from build123d import *

# Parameters (mm, degrees)
SKETCH_R     = 4
PAD_DEPTH    = 8
SKETCH001_R  = 2.85
PAD001_DEPTH = 9
SKETCH002_R  = 2.4
PAD002_DEPTH = 6
CHAMFER_SIZE = 1


with BuildPart() as part:
    # Sketch → Pad (new body)
    with BuildSketch(Plane.XY):
        Circle(SKETCH_R)
    extrude(amount=PAD_DEPTH)

    # Sketch001 (on Face3 of Pad) → Pad001 (join)
    with BuildSketch(Plane.XY.offset(8)):
        Circle(SKETCH001_R)
    extrude(amount=PAD001_DEPTH)

    # Sketch002 (on Face5 of Pad001) → Pad002 (join)
    with BuildSketch(Plane.XY.offset(17)):
        Circle(SKETCH002_R)
    extrude(amount=PAD002_DEPTH)

    # Chamfer
    chamfer_edges = [part.edges().sort_by_distance(p)[0] for p in [
        (-4, 0, 0),
    ]]
    chamfer(chamfer_edges, length=CHAMFER_SIZE)


solid = part.part
Part model, mm, in its own coordinate system. A direction names the side the tool comes from. Coordinates: 2 decimals unless noted, no trailing zeros. Order: outer loops, then holes, each group sorted by start corner. A loop starts at its lowest first (then second) coordinate and runs counter-clockwise, first axis right, second up. Notation, with made-up numbers: M 60.5,20.5 L 99.5,20.5 A22 cw 99.5,46.5 Z; hole C -21,33 d2. An arc over 180 degrees is marked long. Use a Markdown table: item, result.
(1) Probe L1, parallel to Z at x = -2, y = 1.5; L2, parallel to Y at x = -2.5, z = 5; L3, parallel to X at y = 0.5, z = 3. List the from-to ranges inside material, lowest first.
A:
| item | result |
|---|---|
| L1 | z = 0 to 17 |
| L2 | y = -3.12 to 3.12 |
| L3 | x = -3.97 to 3.97 |
(2) Flat gauge pins, fed straight in: pin 1 (4 mm diameter, centred on y = -1.5, z = 17, fed in from -X); pin 2 (3 mm diameter, centred on x = -2, y = 1, fed in from -Z); pin 3 (1 mm diameter, centred on x = 0, y = 3, fed in from +Z). Where does each tip first touch, or does it go through?
A:
| item | result |
|---|---|
| pin 1 | stops at x = -2.85 |
| pin 2 | stops at z = 0 |
| pin 3 | stops at z = 17 |
(3) Cut at A-A on y = 0. Write the cut outline in (x, z), then the cut area to 3 significant figures.
A:
| item | result |
|---|---|
| outline | M -4,1 L -3,0 L 3,0 L 4,1 L 4,8 L 2.85,8 L 2.85,17 L 2.4,17 L 2.4,23 L -2.4,23 L -2.4,17 L -2.85,17 L -2.85,8 L -4,8 Z |
| area | 143 mm^2 |
(4) Cut at D-D on z = 9.25. Write the cut outline in (x, y), then the cut area to 3 significant figures.
A:
| item | result |
|---|---|
| outline | C 0,0 d5.7 |
| area | 25.5 mm^2 |
(5) Tool access for faces 1 (the flat face through (0, 0, 0)), 2 (the cylindrical face through (1.29, 2.024, 19.958)): list every direction of +Z, -Z, +X, -X, +Y, -Y with a clear straight run to the whole face (end or side of a thin tool).
A:
| item | result |
|---|---|
| face 1 | -Z, +X, -X, +Y, -Y |
| face 2 | +Z |
(6) Cut at C-C on z = 5. Write the cut outline in (x, y).
A:
| item | result |
|---|---|
| outline | C 0,0 d8 |
(7) Pull direction X, two halves, no side cores. Call faces 3 (the cylindrical face through (-2.262, -1.734, 12.437)), 4 (the flat face through (-1, 3, 8)): released by +X, released by -X, zero draft, split by the parting line, or undercut.
A:
| item | result |
|---|---|
| face 3 | split by the parting line |
| face 4 | zero draft |
